Design review of the part built by this model. Coordinates are the model's own, in mm. A direction names the side the tool comes from. Give positions to 0.01 mm unless a question says otherwise; leave off trailing zeros. Order: outer loops, then holes, each group sorted by start corner. A loop starts at its lowest first (then second) coordinate and runs counter-clockwise, first axis right, second up. Notation, with made-up numbers: M -8,-6 L 51,-6 A17 ccw 51,0 Z; hole C -27,55 d8. An arc over 180 degrees is marked long. Put each result on its own line as item: value. Start each with the question number.
from build123d import *

# Parameters (mm, degrees)
SKETCH1_R           = 6.25
SKETCH1_R_2         = 4.25
SKETCH1_R_3         = 3.25
SKETCH1_R_4         = 11.5
SKETCH1_R_5         = 1.75
BOSS_EXTRUDE1_DEPTH = 3
SKETCH2_W           = 50
SKETCH2_H           = 50
SKETCH2_R           = 11.5
SKETCH2_R_2         = 1.75
BOSS_EXTRUDE2_DEPTH = 3
CHAMFER1_SIZE       = 10
CHAMFER2_SIZE       = 30


with BuildPart() as part:
    # Sketch1 → Boss-Extrude1 (new body)
    with BuildSketch(Plane(origin=(0, 0, 0), x_dir=(1, 0, 0), z_dir=(0, 1, 0))):
        Polygon((-245, 230), (295, 230), (295, -230), (-295, -230), (-295, 230), (-295, 280), (-245, 280), align=None)
        with Locations(Location((-140, 210, 0), (0, 0, 270))):
            Circle(SKETCH1_R, mode=Mode.SUBTRACT)
        with Locations(Location((140, 210, 0), (0, 0, 270))):
            Circle(SKETCH1_R, mode=Mode.SUBTRACT)
        with Locations(Location((-180, 110, 0), (0, 0, 270))):
            Circle(SKETCH1_R_2, mode=Mode.SUBTRACT)
        with Locations(Location((180, 110, 0), (0, 0, 270))):
            Circle(SKETCH1_R_2, mode=Mode.SUBTRACT)
        with Locations(Location((243.695652174, 220, 0), (0, 0, 270))):
            Circle(SKETCH1_R_3, mode=Mode.SUBTRACT)
        with Locations(Location((282.173913043, 220, 0), (0, 0, 270))):
            Circle(SKETCH1_R_3, mode=Mode.SUBTRACT)
        with Locations(Location((282.173913043, 190, 0), (0, 0, 270))):
            Circle(SKETCH1_R_3, mode=Mode.SUBTRACT)
        with Locations(Location((243.695652174, 190, 0), (0, 0, 270))):
            Circle(SKETCH1_R_3, mode=Mode.SUBTRACT)
        with Locations(Location((-282.173913043, 220, 0), (0, 0, 90))):
            Circle(SKETCH1_R_3, mode=Mode.SUBTRACT)
        with Locations(Location((-243.695652174, 220, 0), (0, 0, 90))):
            Circle(SKETCH1_R_3, mode=Mode.SUBTRACT)
        with Locations(Location((-243.695652174, 190, 0), (0, 0, 90))):
            Circle(SKETCH1_R_3, mode=Mode.SUBTRACT)
        with Locations(Location((-282.173913043, 190, 0), (0, 0, 90))):
            Circle(SKETCH1_R_3, mode=Mode.SUBTRACT)
        with Locations(Location((-270, 255, 0), (0, 0, 270))):
            Circle(SKETCH1_R_4, mode=Mode.SUBTRACT)
        with Locations(Location((-285.5, 239.5, 0), (0, 0, 270))):
            Circle(SKETCH1_R_5, mode=Mode.SUBTRACT)
        with Locations(Location((-285.5, 270.5, 0), (0, 0, 270))):
            Circle(SKETCH1_R_5, mode=Mode.SUBTRACT)
        with Locations(Location((-254.5, 270.5, 0), (0, 0, 270))):
            Circle(SKETCH1_R_5, mode=Mode.SUBTRACT)
        with Locations(Location((-254.5, 239.5, 0), (0, 0, 270))):
            Circle(SKETCH1_R_5, mode=Mode.SUBTRACT)
        with BuildLine():
            Line((-180, 180), (180, 180))
            Line((180, 180), (180, 121.25))
            ThreePointArc((180, 121.25), (168.75, 110), (180, 98.75))
            Line((180, 98.75), (245, 60))
            Line((245, 60), (245, -180))
            Line((245, -180), (-245, -180))
            Line((-245, -180), (-245, 60))
            Line((-245, 60), (-180.004119379, 98.750000754))
            ThreePointArc((-180.004119379, 98.750000754), (-168.750000189, 109.997940311), (-180, 121.25))
            Line((-180, 121.25), (-180, 180))
        make_face(mode=Mode.SUBTRACT)
    extrude(amount=BOSS_EXTRUDE1_DEPTH)

    # Sketch2 → Boss-Extrude2 (add)
    with BuildSketch(Plane(origin=(0, 3, 0), x_dir=(1, 0, 0), z_dir=(0, 1, 0))):
        with Locations((270, 255)):
            Rectangle(SKETCH2_W, SKETCH2_H)
        with Locations(Location((270, 255, 0), (0, 0, 270))):
            Circle(SKETCH2_R, mode=Mode.SUBTRACT)
        with Locations(Location((254.5, 270.5, 0), (0, 0, 270))):
            Circle(SKETCH2_R_2, mode=Mode.SUBTRACT)
        with Locations(Location((285.5, 270.5, 0), (0, 0, 270))):
            Circle(SKETCH2_R_2, mode=Mode.SUBTRACT)
        with Locations(Location((254.5, 239.5, 0), (0, 0, 270))):
            Circle(SKETCH2_R_2, mode=Mode.SUBTRACT)
        with Locations(Location((285.5, 239.5, 0), (0, 0, 270))):
            Circle(SKETCH2_R_2, mode=Mode.SUBTRACT)
    extrude(amount=-BOSS_EXTRUDE2_DEPTH)

    # Chamfer1
    chamfer1_edges = [part.edges().sort_by_distance(p)[0] for p in [
        (-295, 1.5, -280),
        (-245, 1.5, -280),
        (-245, 1.5, -230),
        (245, 1.5, -280),
        (245, 1.5, -230),
        (295, 1.5, -280),
    ]]
    chamfer(chamfer1_edges, length=CHAMFER1_SIZE)

    # Chamfer2
    chamfer2_edges = [part.edges().sort_by_distance(p)[0] for p in [
        (295, 1.5, 230),
        (-295, 1.5, 230),
        (245, 1.5, 180),
        (-245, 1.5, 180),
    ]]
    chamfer(chamfer2_edges, length=CHAMFER2_SIZE)


solid = part.part
1. Machinability: for faces 4 (the flat face through (-280, 1, 215)), 5 (the flat face through (-212.96, 1.48, -79.1)), which of the approach directions +Z, -Z, +X, -X, +Y, -Y give a long, thin tool a straight path to every point of the face, cutting with its end or side? Answer none if there is none.
2. The part is to be moulded in two halves that separate along X. For faces 1 (the flat face through (-4, 0, -199)), 2 (the cylindrical face through (-280.2, 1.48, -249.69)), 3 (the flat face through (280, 1, 215)), say which applies: +X half, -X half, draft (parallel to the pull), parting line (faces both ways), or undercut.
3. Consider section D-D on z = 7. Give the boundary of the cut face in (x, y), then the cut area to 3 significant figures.
4. Consider section C-C on x = 14. Give the boundary of the cut face in (y, z), then the cut area to 3 significant figures.
5. Consider section A-A on x = -140. Give the boundary of the cut face in (y, z).
6. To check wall thickness, follow probe 1 along X at (y, z) = (1.8, -60); probe 2 along X at (y, z) = (2.2, -255); probe 3 along Z at (x, y) = (71, 0.6). State the ranges of each line that lie inside material, in increasing order.
7. Consider section B-B on z = -255. Give the boundary of the cut face in (x, y), then the cut area to 3 significant figures.
Returned:
1. face 4: +Z, -X, +Y, -Y
1. face 5: +Y, -Y
2. face 1: draft
2. face 2: undercut
2. face 3: +X half
3. outline: M -295,0 L -245,0 L -245,3 L -295,3 Z; M 245,0 L 295,0 L 295,3 L 245,3 Z
3. area: 300 mm2
4. outline: M 0,-230 L 3,-230 L 3,-180 L 0,-180 Z; M 0,180 L 3,180 L 3,230 L 0,230 Z
4. area: 300 mm2
5. outline: M 0,-230 L 3,-230 L 3,-216.25 L 0,-216.25 Z; M 0,-203.75 L 3,-203.75 L 3,-180 L 0,-180 Z; M 0,180 L 3,180 L 3,230 L 0,230 Z
6. probe 1: x = -295 to -245, 245 to 295
6. probe 2: x = -295 to -281.5, -258.5 to -245, 245 to 258.5, 281.5 to 295
6. probe 3: z = -230 to -180, 180 to 230
7. outline: M -295,0 L -281.5,0 L -281.5,3 L -295,3 Z; M -258.5,0 L -245,0 L -245,3 L -258.5,3 Z; M 245,0 L 258.5,0 L 258.5,3 L 245,3 Z; M 281.5,0 L 295,0 L 295,3 L 281.5,3 Z
7. area: 162 mm2
